from build123d import *

# Parameters (mm, degrees)
F0_R     = 3.5
F1_DEPTH = 5
F3_DEPTH = 1.5


with BuildPart() as f1:
    # F0 (on Top) → F1 (new body)
    with BuildSketch(Plane.XY):
        Circle(F0_R)
    extrude(amount=-F1_DEPTH)

    # F2 (on Top) → F3 (join)
    with BuildSketch(Plane.XY):
        with BuildLine():
            Line((3, 1.802776), (2, 14.64963))
            ThreePointArc((2, 14.64963), (0, 16.5), (-2, 14.64963))
            Line((-2, 14.64963), (-3, 1.802776))
            ThreePointArc((-3, 1.802776), (0, 3.5), (3, 1.802776))
        make_face()
    extrude(amount=-F3_DEPTH)


solid = f1.part
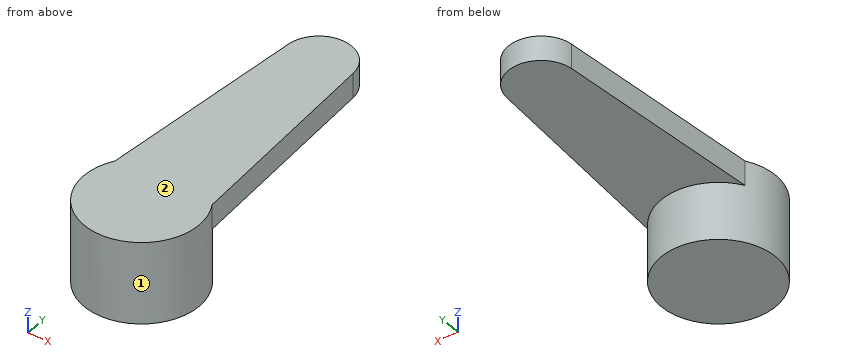
The listing builds one solid part. Answer for the finished solid, in the listing's coordinates (mm). Face numbers are marked on the shaded views. A direction names the side the tool comes from. Coordinates: 2 decimals unless noted, no trailing zeros. Write each loop counter-clockwise with the first axis right and the second up, starting at its lowest first coordinate (ties: lowest second). Pieces come first, ordered by that corner, then holes. Notation, with made-up numbers: M 41.5,54.5 L 66.5,54.5 A27 ccw 66.5,91.5 Z; hole C -27.75,-23 d6. An arc over 180 degrees is marked long. Use one line per item in the form item = value.
Item 1: Find the intervals of material crossed by probe 1 along Z at (x, y) = (1, 9); probe 2 along Y at (x, z) = (0, -2.2); probe 3 along Y at (x, z) = (-1.75, -0.2), in increasing order.
Model answer:
probe_1 = -1.5 to 0
probe_2 = -3.5 to 3.5
probe_3 = -3.03 to 15.47
Item 2: Find section D-D, the plane x = 2.25. Give the vertices of the cut face in (y, z), plus the area to 3 significant figures.
Model answer:
outline = M -2.68,-5 L 2.68,-5 L 2.68,-1.5 L 11.44,-1.5 L 11.44,0 L -2.68,0 Z
area = 39.9 mm2
Item 3: For the marked faces 1 and 2, determine the directions among +Z, -Z, +X, -X, +Y, -Y from which every point of the face is accessible in a straight line to the end or side of a thin tool.
Model answer:
face_1 = -Z
face_2 = +Z, +X, -X, +Y, -Y
Item 4: Find section C-C, the plane y = 13. Give the vertices of the cut face in (x, z), plus the area to 3 significant figures.
Model answer:
outline = M -2.13,-1.5 L 2.13,-1.5 L 2.13,0 L -2.13,0 Z
area = 6.39 mm2
Item 5: Find section A-A, the plane x = 0. Give the vertices of the cut face in (y, z).
Model answer:
outline = M -3.5,-5 L 3.5,-5 L 3.5,-1.5 L 16.5,-1.5 L 16.5,0 L -3.5,0 Z
Item 6: Given P1, Ø1.5, axis at x = 2.5, y = 1, coming from the +Z side; P2, Ø1, axis at x = 0.5, z = -3, coming from the +Y side; P3, Ø1, axis at x = 0.5, y = 9.5, coming from the -Z side, each flat-ended and moving along its own axis, determine where each tip first touches the part or whether it passes through.
Model answer:
P1 = 0
P2 = 3.5
P3 = -1.5
Item 7: Find section B-B, the plane z = -1.95. Give the vertices of the cut face in (x, y).
Model answer:
outline = C 0,0 d7
